```python
from build123d import *

# Parameters (mm, degrees)
SKETCH1_R           = 1.5
BOSS_EXTRUDE1_DEPTH = 50
SKETCH2_R           = 3.001667429
BOSS_EXTRUDE2_DEPTH = 11.7
BOSS_EXTRUDE2_DRAFT = -3
BOSS_EXTRUDE3_DEPTH = 17
SKETCH10_W          = 12
SKETCH10_H          = 4.3
BOSS_EXTRUDE4_DEPTH = 12
SKETCH11_W          = 11.6
SKETCH11_H          = 2.5
CUT_EXTRUDE1_DEPTH  = 12
SKETCH12_W          = 2.5
SKETCH12_H          = 2
CUT_EXTRUDE2_DEPTH  = 0.5
SKETCH14_W          = 2.5
SKETCH14_H          = 2
CUT_EXTRUDE4_DEPTH  = 0.5
SKETCH16_RX         = 0.950654257
SKETCH16_RY         = 0.480988828
CUT_EXTRUDE5_DEPTH  = 0.5
CUT_EXTRUDE5_TAPER  = 22


with BuildPart() as part:
    # Sketch1 → Boss-Extrude1 (new body)
    with BuildSketch(Plane(origin=(0, 0, 0), x_dir=(1, 0, 0), z_dir=(0, 1, 0))):
        with Locations(Location((0, 0, 0), (0, 0, 270))):
            Circle(SKETCH1_R)
    extrude(amount=BOSS_EXTRUDE1_DEPTH)


with BuildPart() as boss_extrude2_tool:
    # Sketch2 → Boss-Extrude2 (with draft: the straight prism first)
    with BuildSketch(Plane(origin=(0, 50, 0), x_dir=(1, 0, 0), z_dir=(0, 1, 0))):
        Circle(SKETCH2_R)
    extrude(amount=BOSS_EXTRUDE2_DEPTH)
    # Boss-Extrude2: the draft: its side faces are tilted about the plane it starts from
    boss_extrude2_sides = [boss_extrude2_tool.faces().sort_by_distance(p)[0] for p in [
        (-3.001667429, 55.85, 0),
    ]]
    draft(boss_extrude2_sides, Plane(origin=(0, 50, 0), x_dir=(1, 0, 0), z_dir=(0, 1, 0)), BOSS_EXTRUDE2_DRAFT)


with BuildPart() as part_1:
    add(part.part)

    # Boss-Extrude2: add boss_extrude2_tool
    add(boss_extrude2_tool.part)

    # Sketch9 → Boss-Extrude3 (add)
    with BuildSketch(Plane(origin=(0, 61.7, 0), x_dir=(1, 0, 0), z_dir=(0, 1, 0))):
        with BuildLine():
            ThreePointArc((-7.2, 3.614838447), (0, 4.114838447), (7.2, 3.614838447))
            ThreePointArc((7.2, 3.614838447), (7.7, 0), (7.2, -3.614838447))
            ThreePointArc((7.2, -3.614838447), (0, -4.114838447), (-7.2, -3.614838447))
            ThreePointArc((-7.2, -3.614838447), (-7.7, 0), (-7.2, 3.614838447))
        make_face()
    extrude(amount=BOSS_EXTRUDE3_DEPTH)

    # Sketch10 → Boss-Extrude4 (add)
    with BuildSketch(Plane(origin=(0, 78.7, 0), x_dir=(1, 0, 0), z_dir=(0, 1, 0))):
        Rectangle(SKETCH10_W, SKETCH10_H)
    extrude(amount=BOSS_EXTRUDE4_DEPTH)

    # Sketch11 → Cut-Extrude1 (cut)
    with BuildSketch(Plane(origin=(0, 90.7, 0), x_dir=(1, 0, 0), z_dir=(0, 1, 0))):
        with Locations((0, 0.7)):
            Rectangle(SKETCH11_W, SKETCH11_H)
    extrude(amount=-CUT_EXTRUDE1_DEPTH, mode=Mode.SUBTRACT)

    # Sketch12 → Cut-Extrude2 (cut)
    with BuildSketch(Plane.XY.offset(2.15)):
        with Locations((-2.75, 84.7)):
            Rectangle(SKETCH12_W, SKETCH12_H)
        with Locations((2.75, 84.7)):
            Rectangle(SKETCH12_W, SKETCH12_H)
    extrude(amount=-CUT_EXTRUDE2_DEPTH, mode=Mode.SUBTRACT)

    # Sketch14 → Cut-Extrude4 (cut)
    with BuildSketch(Plane(origin=(0, 0, -2.15), x_dir=(-1, 0, 0), z_dir=(0, 0, -1))):
        with Locations((-2.75, 84.7)):
            Rectangle(SKETCH14_W, SKETCH14_H)
        with Locations((2.75, 84.7)):
            Rectangle(SKETCH14_W, SKETCH14_H)
    extrude(amount=-CUT_EXTRUDE4_DEPTH, mode=Mode.SUBTRACT)

    # Sketch16 → Cut-Extrude5 (cut)
    with BuildSketch(Plane(origin=(0, 0, -2.15), x_dir=(-1, 0, 0), z_dir=(0, 0, -1))):
        with Locations((0, 80.942553869)):
            Ellipse(SKETCH16_RX, SKETCH16_RY)
    extrude(amount=-CUT_EXTRUDE5_DEPTH, taper=CUT_EXTRUDE5_TAPER, mode=Mode.SUBTRACT)


solid = part_1.part
```
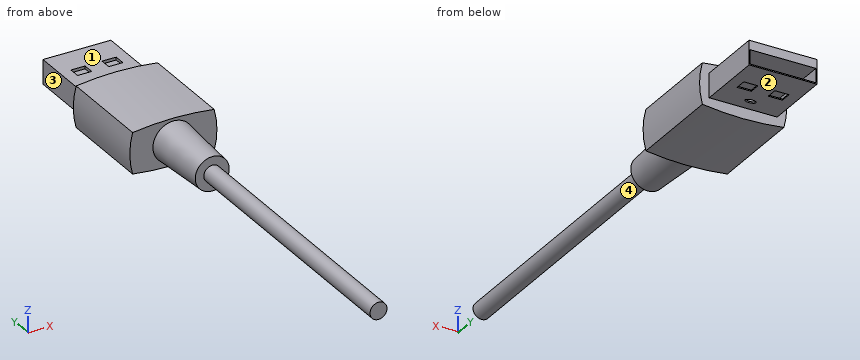
CAD build for the part. Positions are in the model's coordinates, mm. Face numbers are marked on the shaded views. A direction names the side the tool comes from. Coordinates: 2 decimals unless noted, no trailing zeros. Order: outer loops, then holes, each group sorted by start corner. A loop starts at its lowest first (then second) coordinate and runs counter-clockwise, first axis right, second up. Notation, with made-up numbers: M 39,-13 L 74,-13 A23 ccw 74,9 Z; hole C -1,48 d2. An arc over 180 degrees is marked long. Answer as CSV lines item,"result".
1) Cut at A-A (y = 27.5). List the corners of the cut face in (x, z).
Verdict:
outline,"C 0,0 d3"
2) Drill centre lines: L1, parallel to Z at x = 0, y = 85.5; L2, parallel to Y at x = 0, z = -1.75; L3, parallel to Y at x = 3.75, z = -2.5. Where is each one in solid material? Low to high. Write a range as from..to.
Verdict:
L1,"-2.15..-1.95, 0.55..2.15"
L2,"50..78.7"
L3,"61.7..78.7"
3) 3-axis set-ups, long thin cutter, end or side, ignore diameter. For the marked faces 1, 2, 3 and 4: which of +Z, -Z, +X, -X, +Y, -Y reach the whole face in a straight line?
Verdict:
face 1,"+Z, +X, -X, +Y"
face 2,"-Z, +X, -X, +Y"
face 3,"+Z, -Z, -X, +Y"
face 4,"-Y"
4) Flat gauge pins, fed straight in: P1, Ø3, axis at y = 82, z = -1, coming from the +X side; P2, Ø1.5, axis at y = 29.5, z = -1.5, coming from the +X side; P3, Ø2, axis at y = 30, z = -2, coming from the +X side; P4, Ø3, axis at x = -0.5, z = -1.5, coming from the +Y side. Where does each tip first touch, or does it go through?
Verdict:
P1,"x = 6"
P2,"x = 1.3"
P3,"x = 1.12"
P4,"y = 90.7"
